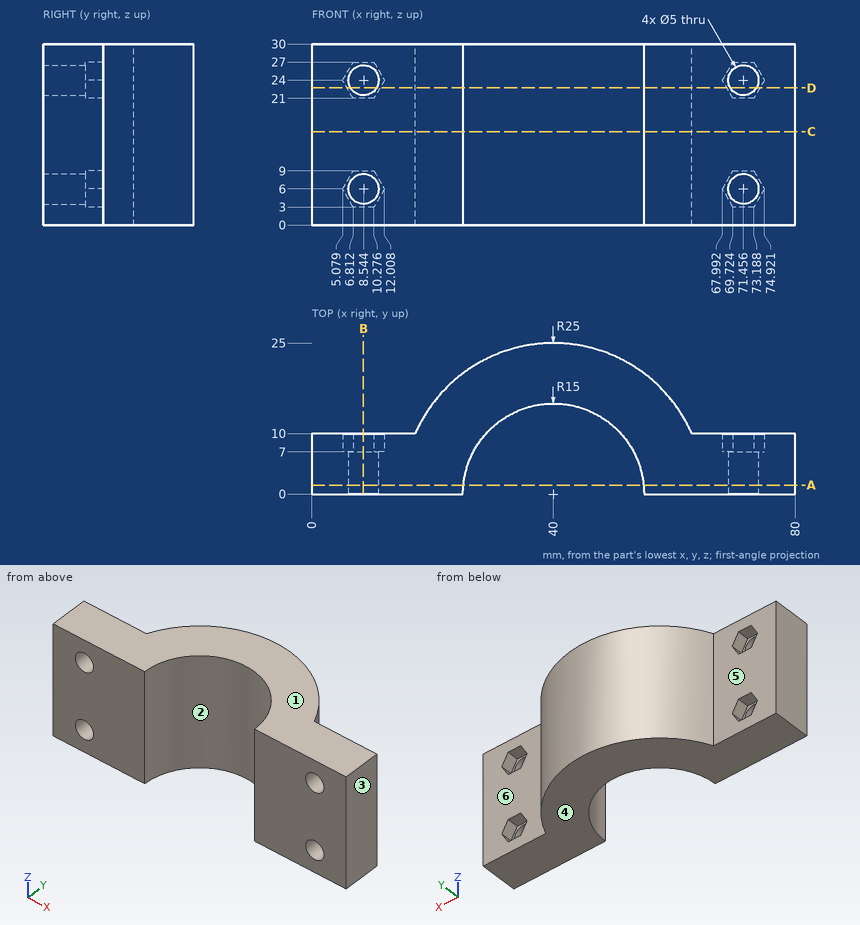
Source: three-view drawing plus pictorial views. Frame: mm from the lowest corner of the part. A direction names the side the tool comes from. Round coordinates to 2 decimals unless told otherwise and drop trailing zeros. Write each loop counter-clockwise with the first axis right and the second up, starting at its lowest first coordinate (ties: lowest second). Pieces come first, ordered by that corner, then holes. Notation, with made-up numbers: M -18.75,-18 L 13.25,-18 A28 ccw 13.25,6 Z; hole C -16.75,20.5 d10. An arc over 180 degrees is marked long. One line per item, written item: value. Start each with the question number.
Item 1: Set-up query: the marked faces 4, 5 and 6. Return all of +Z, -Z, +X, -X, +Y, -Y with unobstructed straight access to the full face (end or side cutting, diameter ignored); none if empty.
Item 2: Pin query (flat end, axial travel): pin 1 (5 mm diameter, centred on x = 9, z = 11.5, fed in from +Y); pin 2 (3 mm diameter, centred on x = 25.5, z = 7, fed in from +Y) (1 decimal); pin 3 (8 mm diameter, centred on y = 21, z = 10.5, fed in from -X). Return the tip coordinate at first contact, or that it passes through.
Item 3: Mould query, pull axis X, two halves, no side actions, for the marked faces 1, 2 and 3. Classes: pulls with the +X half, pulls with the -X half, needs draft (parallel to the pull), parting line crosses it, or undercut.
Item 4: Section query B-B (x = 8.5). Return the cut outline in (y, z).
Item 5: Ray query, L1, parallel to Y at x = 15, z = 3.5; L2, parallel to X at y = 1.75, z = 17; L3, parallel to Y at x = 51.5, z = 13 (1 decimal). Return the intervals inside material, ascending. Write a range as from..to.
Item 6: Section query C-C (z = 15.5). Return the cut outline in (x, y).
Item 7: Section query D-D (z = 22.75). Return the cut outline in (x, y) (1 decimal).
Item 8: Section query A-A (y = 1.5). Return the cut outline in (x, z) (1 decimal), plus the area to 3 significant figures.
Result set:
1. face 4: -Z, +X, -X, +Y, -Y
1. face 5: +Z, -Z, -X, +Y
1. face 6: +Z, -Z, +X, +Y
2. pin 1: stops at y = 10
2. pin 2: stops at y = 21.4
2. pin 3: stops at x = 21.67
3. face 1: needs draft
3. face 2: undercut
3. face 3: pulls with the +X half
4. outline: M 0,0 L 10,0 L 10,3 L 7,3 L 7,3.5 L 0,3.5 Z; M 0,8.5 L 7,8.5 L 7,9 L 10,9 L 10,21 L 7,21 L 7,21.5 L 0,21.5 Z; M 0,26.5 L 7,26.5 L 7,27 L 10,27 L 10,30 L 0,30 Z
5. L1: y = 0..10
5. L2: x = 0..25.1, 54.9..80
5. L3: y = 9.6..22.2
6. outline: M 0,0 L 25,0 A15 cw 55,0 L 80,0 L 80,10 L 62.91,10 A25 ccw 17.09,10 L 0,10 Z
7. outline: M 0,0 L 6.4,0 L 6.4,7 L 5.8,7 L 5.8,10 L 0,10 Z; M 10.7,0 L 25,0 A15 cw 55,0 L 69.3,0 L 69.3,7 L 68.7,7 L 68.7,10 L 62.9,10 A25 ccw 17.1,10 L 11.3,10 L 11.3,7 L 10.7,7 Z; M 73.6,0 L 80,0 L 80,10 L 74.2,10 L 74.2,7 L 73.6,7 Z
8. outline: M 0,0 L 25.1,0 L 25.1,30 L 0,30 Z; M 54.9,0 L 80,0 L 80,30 L 54.9,30 Z; hole C 8.5,6 d5; hole C 8.5,24 d5; hole C 71.5,6 d5; hole C 71.5,24 d5
8. area: 1,430 mm²
